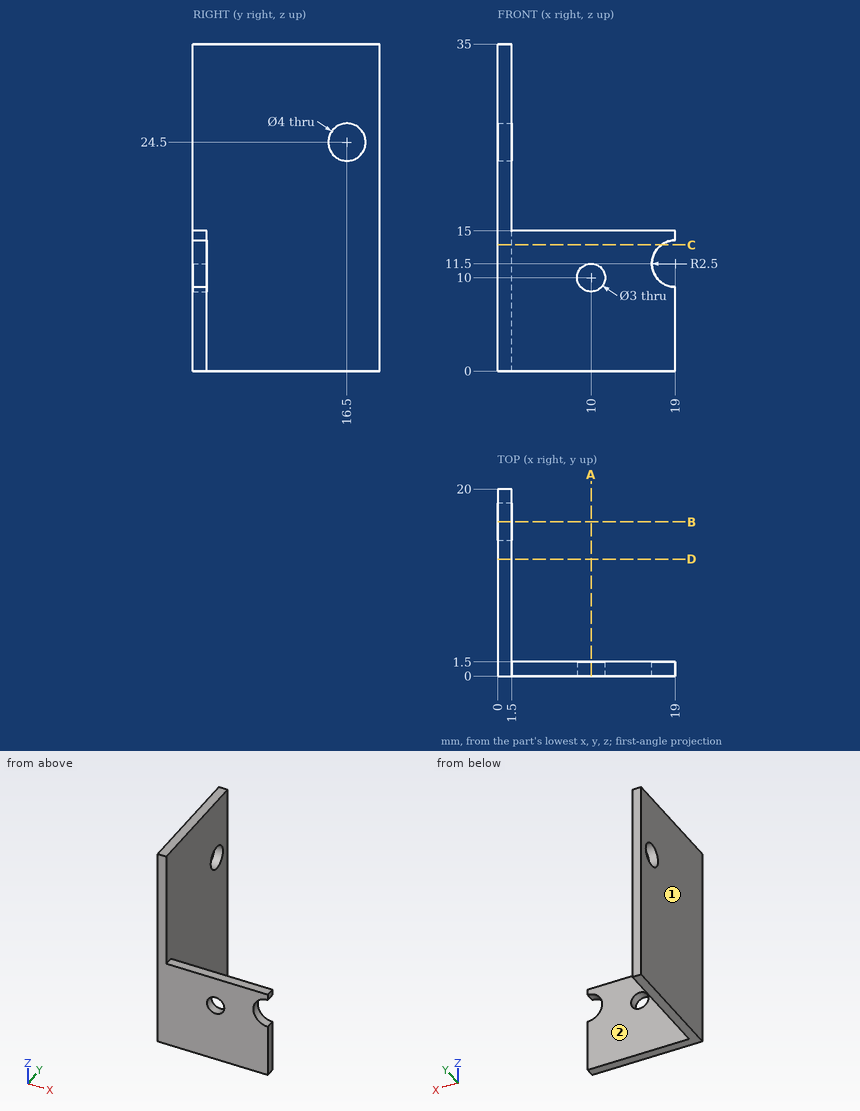
Check sheet for the drawn part. Datum: minimum x, y, z corner. Units: mm. A direction names the side the tool comes from. Coordinates: 2 decimals unless noted, no trailing zeros. Order: outer loops, then holes, each group sorted by start corner. A loop starts at its lowest first (then second) coordinate and runs counter-clockwise, first axis right, second up. Notation, with made-up numbers: (78.25, 78) -> (122.25, 78) arc R9 cw to (122.25, 87) -> close; hole circle Ø9 at (74.25, 1.5). An arc over 180 degrees is marked (long way). Use a Markdown table: item, result. Add a question column.
1. Cross-section at A-A (x = 10). Enter the section's corners in (y, z), and give its area (3 significant figures).
2. Cross-section at C-C (z = 13.5). Enter the section's corners in (x, y), and give its area (3 significant figures).
3. Material ranges on L1, parallel to Z at x = 1, y = 16.5; L2, parallel to Z at x = 10, y = 0.35; L3, parallel to X at y = 17.75, z = 28.5, recorded low to high.
4. Cross-section at B-B (y = 16.5). Enter the section's corners in (x, z), and give its area (3 significant figures).
5. Set-up check for the marked faces 1 and 2: record each of +Z, -Z, +X, -X, +Y, -Y from which the full face is reachable in a straight line by a thin tool's end or side.
6. Cross-section at D-D (y = 12.5). Enter the section's corners in (x, z), and give its area (3 significant figures).
7. Go/stop test with flat-tipped pins: pin 1 Ø4 at (x, y) = (4.5, 8) entering from -Z; pin 2 Ø4 at (x, y) = (2, 7) entering from -Z; pin 3 Ø1 at (y, z) = (5.5, 11) entering from +X; pin 4 Ø3.5 at (x, z) = (10, 10) entering from +Y. Record where each tip stops, or that it passes through.
Filled sheet:
| question | item | result |
|---|---|---|
| 1 | outline | (0, 0) -> (1.5, 0) -> (1.5, 8.5) -> (0, 8.5) -> close; (0, 11.5) -> (1.5, 11.5) -> (1.5, 15) -> (0, 15) -> close |
| 1 | area | 18.0 mm2 |
| 2 | outline | (0, 0) -> (17.5, 0) -> (17.5, 1.5) -> (1.5, 1.5) -> (1.5, 20) -> (0, 20) -> close |
| 2 | area | 54.0 mm2 |
| 3 | L1 | 0 to 22.5, 26.5 to 35 |
| 3 | L2 | 0 to 8.5, 11.5 to 15 |
| 3 | L3 | 0 to 1.5 |
| 4 | outline | (0, 0) -> (1.5, 0) -> (1.5, 22.5) -> (0, 22.5) -> close; (0, 26.5) -> (1.5, 26.5) -> (1.5, 35) -> (0, 35) -> close |
| 4 | area | 46.5 mm2 |
| 5 | face 1 | +Z, -Z, -X, +Y, -Y |
| 5 | face 2 | +Z, -Z, +X, +Y |
| 6 | outline | (0, 0) -> (1.5, 0) -> (1.5, 35) -> (0, 35) -> close |
| 6 | area | 52.5 mm2 |
| 7 | pin 1 | through |
| 7 | pin 2 | z = 0 |
| 7 | pin 3 | x = 1.5 |
| 7 | pin 4 | y = 1.5 |
